from build123d import *

# Parameters (mm, degrees)
F0_W     = 81.3596632027
F0_H     = 50
F1_DEPTH = 25
F2_T     = 2.5


with BuildPart() as f1:
    # F0 (on Front) → F1 (new body)
    with BuildSketch(Plane.XZ):
        with Locations((40.6798316013, 25)):
            Rectangle(F0_W, F0_H)
    extrude(amount=F1_DEPTH)

    # F2
    f2_openings = [f1.faces().sort_by_distance(p)[0] for p in [
        (40.679832, -25, 25),
    ]]
    offset(amount=F2_T, openings=f2_openings, kind=Kind.INTERSECTION)


solid = f1.part
Verification items for the finished model (mm, model axes). A direction names the side the tool comes from. Round coordinates to 2 decimals unless told otherwise and drop trailing zeros. Order: outer loops, then holes, each group sorted by start corner. A loop starts at its lowest first (then second) coordinate and runs counter-clockwise, first axis right, second up. Notation, with made-up numbers: (72, 72.25) -> (76, 72.25) arc R15 ccw to (76, 80.25) -> close; hole circle Ø2 at (13.5, -36.75). An arc over 180 degrees is marked (long way). Put each result on its own line as item: value.
1) Material ranges on line 1 (Z direction, x = 36, y = -4.25); line 2 (X direction, y = -18, z = 36.5); line 3 (Y direction, x = 23.5, z = 41), recorded low to high.
Final values:
line 1: z = -2.5 to 0, 50 to 52.5
line 2: x = -2.5 to 0, 81.36 to 83.86
line 3: y = 0 to 2.5
2) Depth check by flat-ended pin: pin 1 (15 mm diameter, centred on x = 54, z = 27, fed in from -Y). Enter the tip coordinate at first touch or a pass-through.
Final values:
pin 1: stops at y = 0
3) Section check C-C (z = 45.5). Record the cut outline in (x, y).
Final values:
outline: (-2.5, -25) -> (0, -25) -> (0, 0) -> (81.36, 0) -> (81.36, -25) -> (83.86, -25) -> (83.86, 2.5) -> (-2.5, 2.5) -> close
4) Mould release check, pull along X, two halves, no side actions. Record for faces 3 (the flat face through (83.86, -11, 25)), 4 (the flat face through (37, -25, -1)), 5 (the flat face through (40, -12, 0)): +X half, -X half, draft (parallel to the pull), parting line (faces both ways), or undercut.
Final values:
face 3: +X half
face 4: draft
face 5: undercut
5) Set-up check for faces 1 (the flat face through (40, 0, 25)), 2 (the flat face through (40, 2.5, 25)): record each of +Z, -Z, +X, -X, +Y, -Y from which the full face is reachable in a straight line by a thin tool's end or side.
Final values:
face 1: -Y
face 2: +Z, -Z, +X, -X, +Y
6) Section check A-A (y = -17.5). Record the cut outline in (x, z), then the cut area to 3 significant figures.
Final values:
outline: (-2.5, -2.5) -> (83.86, -2.5) -> (83.86, 52.5) -> (-2.5, 52.5) -> close; hole (0, 0) -> (81.36, 0) -> (81.36, 50) -> (0, 50) -> close
area: 682 mm^2
7) Section check B-B (x = 61). Record the cut outline in (y, z).
Final values:
outline: (-25, -2.5) -> (2.5, -2.5) -> (2.5, 52.5) -> (-25, 52.5) -> (-25, 50) -> (0, 50) -> (0, 0) -> (-25, 0) -> close
